The model under review builds one solid part; all positions refer to its coordinate system, in mm. A direction names the side the tool comes from. Coordinates: 2 decimals unless noted, no trailing zeros. Loops run counter-clockwise (first coordinate to the right, second up) from the corner with the lowest first, then second, coordinate; pieces in that order, holes last. Notation, with made-up numbers: (66, 70) - (79, 70) arc R31 cw to (79, 101) - close; hole circle Ø10 at (81, 57). An arc over 180 degrees is marked (long way). Use a Markdown table: item, result. Add a question column.
1) To check wall thickness, follow L1, parallel to X at y = 1, z = 1.55; L2, parallel to Y at x = 0, z = 2.45; L3, parallel to Y at x = -9, z = 1. State the ranges of each line that lie inside material, in increasing order. Write a range as [from, to].
2) Add section D-D, the plane y = -9. Give the boundary of the cut face in (x, z), and give its area (3 significant figures).
3) Add section A-A, the plane y = 0. Give the boundary of the cut face in (x, z), and give its area (3 significant figures).
4) Add section B-B, the plane x = 0. Give the boundary of the cut face in (y, z), and give its area (3 significant figures).
5) Clearance check with a flat-ended pin moving along its axis: pin 1 (5 mm diameter, centred on x = 0, y = -9, fed in from -Z). State where the tip first meets the part, or that it passes through.
6) The part is to be moulded in two halves that separate along Y. For faces 3 (the cylindrical face through (-11.99, 0.53, 1.48)), 4 (the cylindrical face through (7.8, -0.9, 1.5)), 5 (the flat face through (0, 3, 0)), say which applies: pulls with the +Y half, pulls with the -Y half, needs draft (parallel to the pull), parting line crosses it, or undercut.
7) Add section C-C, the plane z = 2.25. Give the boundary of the cut face in (x, y), and give its area (3 significant figures).
8) For faces 1 (the flat face through (0, 3, 3)), 2 (the flat face through (0, 2.1, 1)), list the 3-axis set-ups (+Z, -Z, +X, -X, +Y, -Y) from which the entire face can be reached by the end or side of a thin tool; tool diameter is ignored.
```python
from build123d import *

# Parameters (mm, degrees)
CROQUIS1_R              = 12
CROQUIS1_R_2            = 1.5
SALIENTE_EXTRUIR1_DEPTH = 3


with BuildPart() as part:
    # Croquis1 → Saliente-Extruir1 (new body)
    with BuildSketch(Plane.XY):
        Circle(CROQUIS1_R)
        with Locations((0, 9)):
            Circle(CROQUIS1_R_2, mode=Mode.SUBTRACT)
        with Locations((9, 0)):
            Circle(CROQUIS1_R_2, mode=Mode.SUBTRACT)
        with Locations((0, -9)):
            Circle(CROQUIS1_R_2, mode=Mode.SUBTRACT)
        with Locations((-9, 0)):
            Circle(CROQUIS1_R_2, mode=Mode.SUBTRACT)
        with BuildLine():
            Line((1.356465997, 2.1), (-1.356465997, 2.1))
            ThreePointArc((-1.356465997, 2.1), (0, -2.5), (1.356465997, 2.1))
        make_face(mode=Mode.SUBTRACT)
    extrude(amount=SALIENTE_EXTRUIR1_DEPTH)


solid = part.part
```
From the geometry:
| question | item | result |
|---|---|---|
| 1 | L1 | x = [-11.96, -10.12], [-7.88, -2.29], [2.29, 7.88], [10.12, 11.96] |
| 1 | L2 | y = [-12, -10.5], [-7.5, -2.5], [2.1, 7.5], [10.5, 12] |
| 1 | L3 | y = [-7.94, -1.5], [1.5, 7.94] |
| 2 | outline | (-7.94, 0) - (-1.5, 0) - (-1.5, 3) - (-7.94, 3) - close; (1.5, 0) - (7.94, 0) - (7.94, 3) - (1.5, 3) - close |
| 2 | area | 38.6 mm^2 |
| 3 | outline | (-12, 0) - (-10.5, 0) - (-10.5, 3) - (-12, 3) - close; (-7.5, 0) - (-2.5, 0) - (-2.5, 3) - (-7.5, 3) - close; (2.5, 0) - (7.5, 0) - (7.5, 3) - (2.5, 3) - close; (10.5, 0) - (12, 0) - (12, 3) - (10.5, 3) - close |
| 3 | area | 39.0 mm^2 |
| 4 | outline | (-12, 0) - (-10.5, 0) - (-10.5, 3) - (-12, 3) - close; (-7.5, 0) - (-2.5, 0) - (-2.5, 3) - (-7.5, 3) - close; (2.1, 0) - (7.5, 0) - (7.5, 3) - (2.1, 3) - close; (10.5, 0) - (12, 0) - (12, 3) - (10.5, 3) - close |
| 4 | area | 40.2 mm^2 |
| 5 | pin 1 | stops at z = 0 |
| 6 | face 3 | parting line crosses it |
| 6 | face 4 | undercut |
| 6 | face 5 | needs draft |
| 7 | outline | circle Ø24 at (0, 0); hole circle Ø3 at (-9, 0); hole circle Ø3 at (0, -9); hole circle Ø3 at (0, 9); hole (-1.36, 2.1) arc R2.5 ccw (long way) to (1.36, 2.1) - close; hole circle Ø3 at (9, 0) |
| 7 | area | 405 mm^2 |
| 8 | face 1 | +Z, +X, -X, +Y, -Y |
| 8 | face 2 | +Z, -Z |
